Build history of the part. All positions in model axes, mm. A direction names the side the tool comes from. Coordinates: 2 decimals unless noted, no trailing zeros. Loops run counter-clockwise (first coordinate to the right, second up) from the corner with the lowest first, then second, coordinate; pieces in that order, holes last. Notation, with made-up numbers: (59.5, 72.25) -> (82.5, 72.25) arc R33 ccw to (82.5, 101.25) -> close; hole circle Ø2 at (13, 29.5). An arc over 180 degrees is marked (long way). One line per item, written item: value. Start each with the question number.
```python
from build123d import *

# Parameters (mm, degrees)
F1_DEPTH = 25.4


with BuildPart() as f1:
    # F0 (on Front) → F1 (new body)
    with BuildSketch(Plane.XZ):
        with BuildLine():
            ThreePointArc((-1.5875, 0), (-1.1225320151, 1.1225320151), (0, 1.5875))
            Line((0, 1.5875), (0, 11.2192574161))
            ThreePointArc((0, 11.2192574161), (-7.9332129988, 7.9332129988), (-11.2192574161, 0))
            Line((-11.2192574161, 0), (-1.5875, 0))
        make_face()
        with BuildLine():
            Line((11.2192574161, 0), (1.5875, 0))
            ThreePointArc((1.5875, 0), (0, -1.5875), (-1.5875, 0))
            Line((-1.5875, 0), (-11.2192574161, 0))
            ThreePointArc((-11.2192574161, 0), (-7.9332129988, -7.9332129988), (0, -11.2192574161))
            Line((0, -11.2192574161), (2.1697970219, -11.007439205))
            ThreePointArc((2.1697970219, -11.007439205), (8.6664654935, -7.1248938813), (11.2192574161, 0))
        make_face()
        with BuildLine():
            ThreePointArc((-11.2192574161, 0), (-7.9332129988, 7.9332129988), (0, 11.2192574161))
            Line((0, 11.2192574161), (0, 47.625))
            ThreePointArc((0, 47.625), (-10.2155761082, 51.3485544162), (-15.6389312991, 60.7724639652))
            Line((-15.6389312991, 60.7724639652), (-12.8842582926, 0))
            Line((-12.8842582926, 0), (-11.2192574161, 0))
        make_face()
        with BuildLine():
            Line((0, 47.625), (0, 11.2192574161))
            ThreePointArc((0, 11.2192574161), (1.0900557407, 11.166177298), (2.1697970219, 11.007439205))
            Line((2.1697970219, 11.007439205), (11.9567549914, 10.0520245243))
            Line((11.9567549914, 10.0520245243), (15.4818237673, 59.9887669064))
            ThreePointArc((15.4818237673, 59.9887669064), (9.9064322447, 51.0952337716), (0, 47.625))
        make_face()
        with BuildLine():
            ThreePointArc((2.1697970219, 11.007439205), (8.6664654935, 7.1248938813), (11.2192574161, 0))
            Line((11.2192574161, 0), (11.2471757098, 0))
            Line((11.2471757098, 0), (11.9567549914, 10.0520245243))
            Line((11.9567549914, 10.0520245243), (2.1697970219, 11.007439205))
        make_face()
        with BuildLine():
            Line((11.2471757098, 0), (11.2192574161, 0))
            ThreePointArc((11.2192574161, 0), (8.6664654935, -7.1248938813), (2.1697970219, -11.007439205))
            Line((2.1697970219, -11.007439205), (34.0019449122, -7.8999464061))
            ThreePointArc((34.0019449122, -7.8999464061), (27.8977093115, -5.8790018171), (25.2932425839, 0))
            Line((25.2932425839, 0), (11.2471757098, 0))
        make_face()
        with BuildLine():
            ThreePointArc((-15.6389312991, 60.7724639652), (-10.2155761082, 51.3485544162), (0, 47.625))
            Line((0, 47.625), (0, 61.9125))
            ThreePointArc((0, 61.9125), (-1.5875, 63.5), (0, 65.0875))
            Line((0, 65.0875), (0, 79.375))
            ThreePointArc((0, 79.375), (-9.8977227148, 75.9117166444), (-15.47687934, 67.0329634722))
            Line((-15.47687934, 67.0329634722), (-15.8215583064, 64.8015059575))
            Line((-15.8215583064, 64.8015059575), (-15.6389312991, 60.7724639652))
        make_face()
        with BuildLine():
            Line((0, 61.9125), (0, 47.625))
            ThreePointArc((0, 47.625), (9.9064322447, 51.0952337716), (15.4818237673, 59.9887669064))
            Line((15.4818237673, 59.9887669064), (15.8215583064, 64.8015059575))
            Line((15.8215583064, 64.8015059575), (15.47687934, 67.0329634722))
            ThreePointArc((15.47687934, 67.0329634722), (9.8977227148, 75.9117166444), (0, 79.375))
            Line((0, 79.375), (0, 65.0875))
            ThreePointArc((0, 65.0875), (1.1225320151, 64.6225320151), (1.5875, 63.5))
            ThreePointArc((1.5875, 63.5), (1.1225320151, 62.3774679849), (0, 61.9125))
        make_face()
        with BuildLine():
            Line((11.9567549914, 10.0520245243), (11.2471757098, 0))
            Line((11.2471757098, 0), (25.2932425839, 0))
            ThreePointArc((25.2932425839, 0), (27.8977093115, 5.8790018171), (34.0019449122, 7.8999464061))
            Line((34.0019449122, 7.8999464061), (11.9567549914, 10.0520245243))
        make_face()
        with BuildLine():
            ThreePointArc((0, -11.2192574161), (1.0900557407, -11.166177298), (2.1697970219, -11.007439205))
            Line((2.1697970219, -11.007439205), (0, -11.2192574161))
        make_face()
        with BuildLine():
            ThreePointArc((-15.8215583064, 64.8015059575), (-15.8587167324, 62.7811616306), (-15.6389312991, 60.7724639652))
            Line((-15.6389312991, 60.7724639652), (-15.8215583064, 64.8015059575))
        make_face()
        with BuildLine():
            Line((15.8215583064, 64.8015059575), (15.4818237673, 59.9887669064))
            ThreePointArc((15.4818237673, 59.9887669064), (15.7763997367, 61.7334110985), (15.875, 63.5))
            ThreePointArc((15.875, 63.5), (15.8616339498, 64.1513013458), (15.8215583064, 64.8015059575))
        make_face()
        with BuildLine():
            ThreePointArc((34.0019449122, 7.8999464061), (27.8977093115, 5.8790018171), (25.2932425839, 0))
            ThreePointArc((25.2932425839, 0), (27.8977093115, -5.8790018171), (34.0019449122, -7.8999464061))
            ThreePointArc((34.0019449122, -7.8999464061), (39.109744401, -5.3330332724), (41.1682425839, 0))
            ThreePointArc((41.1682425839, 0), (39.109744401, 5.3330332724), (34.0019449122, 7.8999464061))
        make_face()
        with BuildLine():
            ThreePointArc((34.8182425839, 0), (33.2307425839, -1.5875), (31.6432425839, 0))
            ThreePointArc((31.6432425839, 0), (33.2307425839, 1.5875), (34.8182425839, 0))
        make_face(mode=Mode.SUBTRACT)
        with BuildLine():
            ThreePointArc((-15.47687934, 67.0329634722), (-15.6889419795, 65.9233704967), (-15.8215583064, 64.8015059575))
            Line((-15.8215583064, 64.8015059575), (-15.47687934, 67.0329634722))
        make_face()
        with BuildLine():
            Line((15.47687934, 67.0329634722), (15.8215583064, 64.8015059575))
            ThreePointArc((15.8215583064, 64.8015059575), (15.6889419795, 65.9233704967), (15.47687934, 67.0329634722))
        make_face()
        with BuildLine():
            ThreePointArc((-15.47687934, 67.0329634722), (-9.8977227148, 75.9117166444), (0, 79.375))
            Line((0, 79.375), (0, 100.0221994281))
            ThreePointArc((0, 100.0221994281), (-1.5875, 101.6096994281), (0, 103.1971994281))
            Line((0, 103.1971994281), (0, 104.775))
            ThreePointArc((0, 104.775), (-5.2438523258, 106.3484191644), (-8.755257881, 110.5488555831))
            Line((-8.755257881, 110.5488555831), (-15.47687934, 67.0329634722))
        make_face()
        with BuildLine():
            Line((0, 100.0221994281), (0, 79.375))
            ThreePointArc((0, 79.375), (9.8977227148, 75.9117166444), (15.47687934, 67.0329634722))
            Line((15.47687934, 67.0329634722), (8.755257881, 110.5488555831))
            ThreePointArc((8.755257881, 110.5488555831), (5.2438523258, 106.3484191644), (0, 104.775))
            Line((0, 104.775), (0, 103.1971994281))
            ThreePointArc((0, 103.1971994281), (1.1225320151, 102.7322314432), (1.5875, 101.6096994281))
            ThreePointArc((1.5875, 101.6096994281), (1.1225320151, 100.4871674129), (0, 100.0221994281))
        make_face()
        with BuildLine():
            ThreePointArc((9.525, 114.3), (-1.9146531909, 123.6305802691), (-8.755257881, 110.5488555831))
            ThreePointArc((-8.755257881, 110.5488555831), (-5.2438523258, 106.3484191644), (0, 104.775))
            ThreePointArc((0, 104.775), (5.2438523258, 106.3484191644), (8.755257881, 110.5488555831))
            ThreePointArc((8.755257881, 110.5488555831), (9.3305802691, 112.3853468091), (9.525, 114.3))
        make_face()
        with BuildLine():
            ThreePointArc((3.175, 114.3), (2.2450640303, 112.0549359697), (0, 111.125))
            ThreePointArc((0, 111.125), (-2.2450640303, 116.5450640303), (3.175, 114.3))
        make_face(mode=Mode.SUBTRACT)
    extrude(amount=F1_DEPTH)


solid = f1.part
```
Item 1: Band-saw the part on D-D, the plane z = 77.5. List the corners of the cut face in (x, y).
Item 2: Band-saw the part on A-A, the plane y = -22. Count the separate pieces of the cut face and the enclosed holes in it, and give its area (3 significant figures).
Item 3: Probe probe 1 along Z at (x, y) = (2, -8.75); probe 2 along X at (y, z) = (-8.25, 114.3) (3 decimals); probe 3 along Z at (x, y) = (34.5, -3.75). List the from-to ranges inside material, lowest first.
Item 4: Drop flat-ended pins along their axis: pin 1 Ø3 at (x, y) = (1.5, -13) entering from +Z (3 decimals); pin 2 Ø0.5 at (x, y) = (-11.5, -13.5) entering from -Z; pin 3 Ø10 at (y, z) = (-16.5, 79) entering from +X; pin 4 Ø7.5 at (x, y) = (6.5, -8.5) entering from +Z. Give the stop position or say it passes through.
Item 5: Two-plate mould, pull along X, no slides. Class faces 1 (the face through (13.695, -12.522, 34.671)), 2 (the face through (34.491, -12.522, -0.966)), 3 (the face through (6, 0, 42)): +X half, -X half, draft (parallel to the pull), parting line (faces both ways), or undercut.
Item 6: Band-saw the part on B-B, the plane x = 4.5. List the corners of the cut face in (y, z).
Item 7: Band-saw the part on C-C, the plane x = 14. List the corners of the cut face in (y, z), and give its area (3 significant figures).
Item 8: Tool access for faces 4 (the face through (23.13, -12.52, 8.96)), 5 (the face through (0, -13, 6)), 6 (the face through (6, -25.4, 42)): list every direction of +Z, -Z, +X, -X, +Y, -Y with a clear straight run to the whole face (end or side of a thin tool).
Worked out:
1. outline: (-13.86, -25.4) -> (13.86, -25.4) -> (13.86, 0) -> (-13.86, 0) -> close
2. separate pieces: 1
2. enclosed holes: 5
2. area: 3,700 mm²
3. probe 1: z = -11.04 to 0, 11.04 to 111.83, 116.77 to 123.61
3. probe 2: x = -9.525 to -3.175, 3.175 to 9.525
3. probe 3: z = -7.84 to -0.95, 0.95 to 7.84
4. pin 1: stops at z = 123.825
4. pin 2: stops at z = 0
4. pin 3: stops at x = 14.4
4. pin 4: stops at z = 123.42
5. face 1: +X half
5. face 2: undercut
5. face 3: draft
6. outline: (-25.4, -10.78) -> (0, -10.78) -> (0, 0) -> (-25.4, 0) -> close; (-25.4, 10.28) -> (0, 10.28) -> (0, 122.69) -> (-25.4, 122.69) -> close
7. outline: (-25.4, -9.85) -> (0, -9.85) -> (0, 9.85) -> (-25.4, 9.85) -> close; (-25.4, 39) -> (0, 39) -> (0, 76.59) -> (-25.4, 76.59) -> close
7. area: 1,460 mm²
8. face 4: +X, +Y, -Y
8. face 5: +Y, -Y
8. face 6: +Z, -Z, +X, -X, -Y
